from build123d import *

# Parameters (mm, degrees)
F0_W     = 10.5
F0_H     = 3
F1_DEPTH = 11
F2_DEPTH = 2
F4_DEPTH = 2
F5_R     = 2
F6_DEPTH = 25
F7_R     = 3.4
F7_R_2   = 2
F8_DEPTH = 7


with BuildPart() as f1:
    # F0 (on Front) → F1 (new body)
    with BuildSketch(Plane.XZ):
        with Locations((6.75, -3.5)):
            Rectangle(F0_W, F0_H)
        with BuildLine():
            Line((1.5, 4), (1.5, 5))
            Line((1.5, 5), (-9.5, 5))
            Line((-9.5, 5), (-9.5, 2))
            ThreePointArc((-9.5, 2), (-7.9057595357, 1.1241546177), (-6.3115190715, 2))
            Line((-6.3115190715, 2), (-1.5, 2))
            Line((-1.5, 2), (-1.5, -4))
            Line((-1.5, -4), (-1.5, -5))
            Line((-1.5, -5), (1.5, -5))
            Line((1.5, -5), (1.5, -2))
            Line((1.5, -2), (1.5, 4))
        make_face()
    extrude(amount=F1_DEPTH)

    # F0 (on Front) → F2 (join)
    with BuildSketch(Plane.XZ):
        Polygon((12, -2), (1.5, 5), (1.5, 4), (1.5, -2), align=None)
    extrude(amount=F2_DEPTH)

    # F3 (on face) → F4 (join)
    with BuildSketch(Plane.XZ.offset(11)):
        Polygon((1.5, -2), (12, -2), (1.5, 5), align=None)
    extrude(amount=-F4_DEPTH)

    # F5 (on face) → F6 (cut)
    with BuildSketch(Plane(origin=(0, 0, -5), x_dir=(1, 0, 0), z_dir=(0, 0, -1))):
        with Locations((7.0000002161, 5.5)):
            Circle(F5_R)
    extrude(amount=-F6_DEPTH, mode=Mode.SUBTRACT)

    # F7 (on face) → F8 (join)
    with BuildSketch(Plane.XY.offset(-2)):
        with Locations((7.0000002161, -5.5)):
            Circle(F7_R)
        with Locations((7.0000002161, -5.5)):
            Circle(F7_R_2, mode=Mode.SUBTRACT)
    extrude(amount=F8_DEPTH)

    # F10 (on offset) → F11 (revolve)
    with BuildSketch(Plane.YZ.offset(7)):
        Polygon((-2.1, 5), (-2.1, -2), (-2, -2), (-0.5000002161, -2), align=None)
    revolve(axis=Axis((7, -5.5, 1.7165149804), (0, 0, 1)))


solid = f1.part
Verification items for the finished model (mm, model axes). A direction names the side the tool comes from. Coordinates: 2 decimals unless noted, no trailing zeros. Loops run counter-clockwise (first coordinate to the right, second up) from the corner with the lowest first, then second, coordinate; pieces in that order, holes last. Notation, with made-up numbers: (9.25, 78) -> (41.25, 78) arc R8 ccw to (41.25, 92) -> close; hole circle Ø9 at (63, 35). An arc over 180 degrees is marked (long way). Answer as a JSON object with one key per item and string values. Group by question number.
Item 1: Tool access check on faces 4 (the flat face through (1.5, -5, 1)), 5 (the flat face through (11.5, -2.8, -2)), 6 (the flat face through (-9.5, -5, 4)), 7 (the flat face through (1, -11, 0)), 8 (the flat face through (-4, -5, 2)). Record the directions out of +Z, -Z, +X, -X, +Y, -Y that give a thin tool (end or side, any length) a straight path to the whole face; none if there is none.
Item 2: Scan lines: probe 1 along X at (y, z) = (-6.5, 4.5); probe 2 along Y at (x, z) = (7, -1.5); probe 3 along X at (y, z) = (-5.5, -1.75). Record each from-to range of solid material in increasing order.
Item 3: Sectioned sample at B-B on x = 7. Record the boundary of the cut face in (y, z).
Item 4: Depth check by flat-ended pin: pin 1 (6 mm diameter, centred on y = -6.5, z = -3.5, fed in from -X); pin 2 (5.5 mm diameter, centred on x = -4.5, y = -6.5, fed in from -Z); pin 3 (5 mm diameter, centred on x = -7, y = -5.5, fed in from -Z). Enter the tip coordinate at first touch or a pass-through.
Item 5: Mould release check, pull along Z, two halves, no side actions. Record for faces 1 (the flat face through (12, -5, -4)), 2 (the flat face through (1.8, -5.5, -2)), 3 (the flat face through (5, -4, -5)): +Z half, -Z half, draft (parallel to the pull), parting line (faces both ways), or undercut.
Item 6: Sectioned sample at C-C on z = -1.25. Record the boundary of the cut face in (x, y) (3 decimals), plus the area to 3 significant figures.
Item 7: Sectioned sample at D-D on x = -5.5. Record the boundary of the cut face in (y, z), plus the area to 3 significant figures.
Item 8: Sectioned sample at A-A on z = 4.25. Record the boundary of the cut face in (x, y) (3 decimals), plus the area to 3 significant figures.
Evaluation:
{
 "1": {"face 4": "+Z", "face 5": "+Z, +X", "face 6": "+Z, -Z, -X, +Y, -Y", "face 7": "+Z, -Z, +X, -X, -Y", "face 8": "-Z, +Y, -Y"},
 "2": {"probe 1": "x = -9.5 to 1.5, 3.63 to 5.27, 8.73 to 10.37", "probe 2": "y = -11 to -7.5, -3.5 to 0", "probe 3": "x = -1.5 to 1.5, 2.06 to 5, 9 to 11.94"},
 "3": {"outline": "(-11, -5) -> (-7.5, -5) -> (-7.5, 5) -> (-8.9, 5) -> (-9.74, 1.33) -> (-11, 1.33) -> close; (-3.5, -5) -> (0, -5) -> (0, 1.33) -> (-1.26, 1.33) -> (-2.1, 5) -> (-3.5, 5) -> close"},
 "4": {"pin 1": "stops at x = -1.5", "pin 2": "stops at z = 1.24", "pin 3": "stops at z = 1.12"},
 "5": {"face 1": "draft", "face 2": "+Z half", "face 3": "-Z half"},
 "6": {"outline": "(-1.5, -11) -> (10.875, -11) -> (10.875, -9) -> (10.326, -9) arc R4.829 ccw to (10.326, -2) -> (10.875, -2) -> (10.875, 0) -> (-1.5, 0) -> close; hole (1.5, -9) -> (3.674, -9) arc R4.829 cw to (3.674, -2) -> (1.5, -2) -> close; hole circle Ø4 at (7, -5.5)", "area": "119 mm²"},
 "7": {"outline": "(-11, 2) -> (0, 2) -> (0, 5) -> (-11, 5) -> close", "area": "33.0 mm²"},
 "8": {"outline": "(-9.5, -11) -> (2.625, -11) -> (2.625, -9) -> (1.5, -9) -> (1.5, -2) -> (2.625, -2) -> (2.625, 0) -> (-9.5, 0) -> close; circle Ø7.143 at (7, -5.5); hole circle Ø4 at (7, -5.5)", "area": "153 mm²"}
}
